Source: CAD feature listing. Evaluate the final solid. Frame: model axes, mm. Round coordinates to 2 decimals unless told otherwise and drop trailing zeros. Loops run counter-clockwise (first coordinate to the right, second up) from the corner with the lowest first, then second, coordinate; pieces in that order, holes last.
(1) Section B-B, the plane x = -61.5. Return the cut outline in (y, z), plus the area to 3 significant figures.
(2) Section C-C, the plane z = 3.25. Return the cut outline in (x, y).
(3) Material intervals for probe 1 along Y at (x, z) = (-52.5, 6); probe 2 along Y at (x, z) = (-59.5, 4.5); probe 3 along X at (y, z) = (-46, 1.75), sorted ascending.
(4) Section A-A, the plane y = -34. Return the cut outline in (x, z).
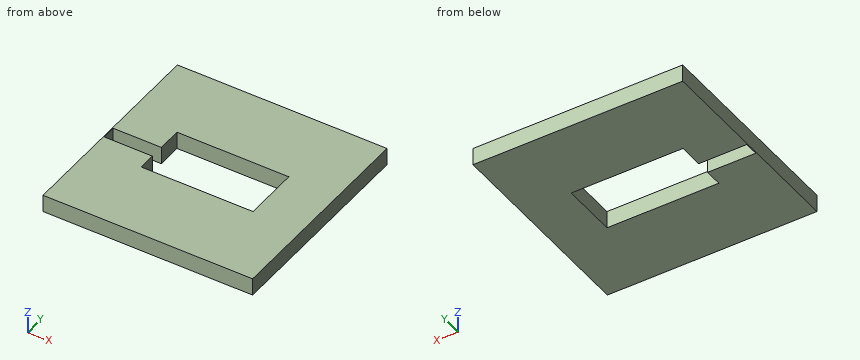
```python
from build123d import *

# Parameters (mm, degrees)
F1_W     = 76.2
F1_H     = 76.2
F1_W_2   = 40.64
F1_H_2   = 20.32
F2_DEPTH = 6.35
F3_W     = 17.763365
F3_H     = 5.08
F4_DEPTH = 25.4


with BuildPart() as f2:
    # F1 (on face) → F2 (new body)
    with BuildSketch(Plane.XY):
        with Locations((-38.1, -38.1)):
            Rectangle(F1_W, F1_H)
        with Locations((-38.1, -38.1)):
            Rectangle(F1_W_2, F1_H_2, mode=Mode.SUBTRACT)
    extrude(amount=F2_DEPTH)

    # F3 (on face) → F4 (cut)
    with BuildSketch(Plane.XY):
        with Locations((-67.033619, -39.375661)):
            Rectangle(F3_W, F3_H)
    extrude(amount=F4_DEPTH, mode=Mode.SUBTRACT)


solid = f2.part
```
Output values:
1. outline: (-76.2, 0) - (-41.92, 0) - (-41.92, 6.35) - (-76.2, 6.35) - close; (-36.84, 0) - (0, 0) - (0, 6.35) - (-36.84, 6.35) - close
1. area: 452 mm2
2. outline: (-76.2, -76.2) - (0, -76.2) - (0, 0) - (-76.2, 0) - close; hole (-75.92, -41.92) - (-58.42, -41.92) - (-58.42, -48.26) - (-17.78, -48.26) - (-17.78, -27.94) - (-58.42, -27.94) - (-58.42, -36.84) - (-75.92, -36.84) - close
3. probe 1: y = -76.2 to -48.26, -27.94 to 0
3. probe 2: y = -76.2 to -41.92, -36.84 to 0
3. probe 3: x = -76.2 to -58.42, -17.78 to 0
4. outline: (-76.2, 0) - (-58.42, 0) - (-58.42, 6.35) - (-76.2, 6.35) - close; (-17.78, 0) - (0, 0) - (0, 6.35) - (-17.78, 6.35) - close
